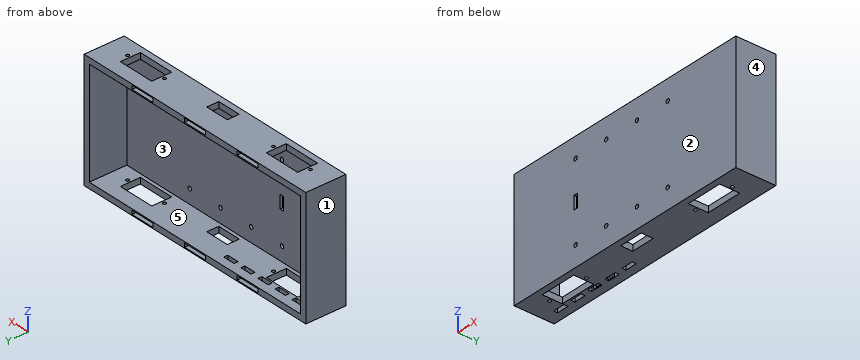
Autodesk Inventor part; units mm, degrees
ref_plane "Work Plane2" through (0, 19.05, 0) normal (0, 1, 0) x (1, 0, 0)
ref_plane "YZ Plane" through (0, 0, 0) normal (1, 0, 0) x (0, 1, 0)
ref_plane "XZ Plane" through (0, 0, 0) normal (0, 1, 0) x (-1, 0, 0)
sketch "Sketch1" plane through (0, 0, 0) normal (0, 1, 0) x (-1, 0, 0)
  line L0 (82.5, 37.5) -> (-82.5, 37.5)
  line L1 (-82.5, 37.5) -> (-82.5, -37.5)
  line L2 (-82.5, -37.5) -> (82.5, -37.5)
  line L3 (82.5, -37.5) -> (82.5, 37.5)
  point P0 (0, 0)
  point P1 (82.5, 0)
  point P2 (0, -37.5)
  dimension "d0" = 165
  dimension "d1" = 75
extrude "Extrusion1" add sketch "Sketch1" along normal blind 25.4
sketch "Sketch2" plane through (-82.5, 0, 37.5) normal (0, 0, 1) x (1, 0, 0)
  line L0 (39.878, 16.51) -> (16.51, 16.51)
  line L1 (39.878, 3.81) -> (39.878, 16.51)
  line L2 (16.51, 3.81) -> (39.878, 3.81)
  line L3 (16.51, 16.51) -> (16.51, 3.81)
  circle A0 centre (14.4272, 10.16) radius 1.016
  circle A1 centre (41.9608, 10.16) radius 1.016
  line L4 (0, 0) -> (165, 0)
  line L5 (0, 0) -> (0, 25.4)
  line L6 (148.49, 16.51) -> (125.122, 16.51)
  circle A2 centre (150.5728, 10.16) radius 1.016
  line L7 (148.49, 3.81) -> (148.49, 16.51)
  line L8 (125.122, 3.81) -> (148.49, 3.81)
  line L9 (125.122, 16.51) -> (125.122, 3.81)
  circle A3 centre (123.0392, 10.16) radius 1.016
  line L10 (165, 0) -> (165, 25.4)
  line L11 (74.88, 11.43) -> (90.12, 11.43)
  line L12 (90.12, 11.43) -> (90.12, 3.81)
  line L13 (90.12, 3.81) -> (74.88, 3.81)
  line L14 (74.88, 3.81) -> (74.88, 11.43)
  point P0 (82.5, 0)
  point P1 (16.51, 10.16)
  point P2 (39.878, 10.16)
  point P3 (0, 12.7)
  point P4 (125.122, 10.16)
  point P5 (82.5, 11.43)
  point P6 (82.5, 0)
  point P7 (74.88, 7.62)
  point P8 (148.49, 10.16)
  point P9 (90.12, 7.62)
  dimension "d4" = 12.7
  dimension "d5" = 23.368
  dimension "d6" = 2.032
  dimension "d7" = 2.032
  dimension "d8" = 2.0828
  dimension "d9" = 2.0828
  dimension "d11" = 16.51
  dimension "d12" = 12.7
  dimension "d13" = 23.368
  dimension "d14" = 2.032
  dimension "d15" = 2.032
  dimension "d16" = 2.0828
  dimension "d17" = 2.0828
  dimension "d18" = 16.51
  dimension "d19" = 15.24
  dimension "d20" = 7.62
  dimension "d55" = 10.16
  dimension "d56" = 10.16
  dimension "d58" = 7.62
extrude "Extrusion2" cut sketch "Sketch2" against normal blind 100.0125
sketch "Sketch3" plane through (0, 25.4, 0) normal (0, 1, 0) x (1, 0, 0)
  line L0 (-78.69, 33.69) -> (78.69, 33.69)
  line L1 (78.69, 33.69) -> (78.69, -33.69)
  line L2 (78.69, -33.69) -> (-78.69, -33.69)
  line L3 (-78.69, -33.69) -> (-78.69, 33.69)
  line L4 (82.5, -37.5) -> (82.5, 37.5)
  line L5 (-82.5, 37.5) -> (-82.5, -37.5)
  line L6 (82.5, 37.5) -> (-82.5, 37.5)
  line L7 (-82.5, -37.5) -> (82.5, -37.5)
  point P0 (0, 0)
  dimension "d25" = 3.81
  dimension "d26" = 3.81
  dimension "d27" = 3.81
  dimension "d28" = 3.81
extrude "Extrusion3" cut sketch "Sketch3" against normal blind 23.8125 contours L0 L1 L2 L3
sketch "Sketch4" plane through (0, 1.5875, 0) normal (0, 1, 0) x (1, 0, 0)
  circle A0 centre (31.7833, 24.6457) radius 1.27
  line L0 (-42.5, 20.5817) -> (42.5, 20.5817)
  circle A1 centre (8.9233, 24.6457) radius 1.27
  circle A2 centre (-13.9367, 24.6457) radius 1.27
  circle A3 centre (-36.7967, 24.6457) radius 1.27
  line L1 (67.3028, 0) -> (-67.3028, 0)
  circle A4 centre (31.7833, -24.6457) radius 1.27
  circle A5 centre (8.9233, -24.6457) radius 1.27
  circle A6 centre (-13.9367, -24.6457) radius 1.27
  circle A7 centre (-36.7967, -24.6457) radius 1.27
  line L2 (78.69, 33.69) -> (78.69, -33.69)
  line L3 (-38.0667, -4.2532) -> (-35.5267, -4.2532)
  line L4 (-35.5267, -4.2532) -> (-35.5267, 4.1493)
  line L5 (-35.5267, 4.1493) -> (-38.0667, 4.1493)
  line L6 (-38.0667, 4.1493) -> (-38.0667, -4.2532)
  point P0 (0, 0)
  point P1 (-11.4746, -1.9183)
  point P2 (78.69, 0)
  point P3 (0, 0)
  point P4 (0, 20.5817)
  point P5 (-36.7967, -4.2532)
  dimension "d35" = 2.54
  dimension "d36" = 4.064
  dimension "d37" = 22.86
  dimension "d159" = 20.3925
  dimension "d160" = 49.2914
extrude "Extrusion4" cut sketch "Sketch4" against normal blind 22.225
ref_plane "Work Plane2" through (0, 19.05, 0) normal (0, 1, 0) x (1, 0, 0)
sketch "Sketch9" plane through (0, 25.4, 0) normal (0, 1, 0) x (1, 0, 0)
  line L0 (-46.8649, 36.8624) -> (-31.3709, 36.8624)
  line L1 (-31.3709, 36.8624) -> (-31.3709, 34.452)
  line L2 (-31.3709, 34.452) -> (-46.8649, 34.452)
  line L3 (-46.8649, 34.452) -> (-46.8649, 36.8624)
  line L4 (31.3709, 36.8624) -> (46.8649, 36.8624)
  line L5 (46.8649, 36.8624) -> (46.8649, 34.452)
  line L6 (46.8649, 34.452) -> (31.3709, 34.452)
  line L7 (31.3709, 34.452) -> (31.3709, 36.8624)
  line L8 (-7.7489, 36.8624) -> (7.7489, 36.8624)
  line L9 (7.7489, 36.8624) -> (7.7489, 34.452)
  line L10 (7.7489, 34.452) -> (-7.7489, 34.452)
  line L11 (-7.7489, 34.452) -> (-7.7489, 36.8624)
  line L12 (82.5, -37.5) -> (82.5, 37.5)
  line L13 (-82.5, 37.5) -> (-82.5, -37.5)
  line L14 (-67.8534, 0) -> (73.4776, 0)
  line L15 (-46.8649, -36.8624) -> (-31.3709, -36.8624)
  line L16 (-31.3709, -36.8624) -> (-31.3709, -34.452)
  line L17 (-31.3709, -34.452) -> (-46.8649, -34.452)
  line L18 (-46.8649, -34.452) -> (-46.8649, -36.8624)
  line L19 (31.3709, -36.8624) -> (46.8649, -36.8624)
  line L20 (46.8649, -36.8624) -> (46.8649, -34.452)
  line L21 (46.8649, -34.452) -> (31.3709, -34.452)
  line L22 (31.3709, -34.452) -> (31.3709, -36.8624)
  line L23 (-7.7489, -36.8624) -> (7.7489, -36.8624)
  line L24 (7.7489, -36.8624) -> (7.7489, -34.452)
  line L25 (7.7489, -34.452) -> (-7.7489, -34.452)
  line L26 (-7.7489, -34.452) -> (-7.7489, -36.8624)
  line L27 (-78.69, 33.69) -> (78.69, 33.69)
  point P0 (0, 0)
  point P1 (-31.3709, 35.6572)
  point P2 (31.3709, 35.6572)
  point P3 (-7.7489, 35.6572)
  point P4 (7.7489, 35.6572)
  point P5 (0, 34.452)
  dimension "d59" = 2.4104
  dimension "d60" = 2.4104
  dimension "d61" = 2.4104
  dimension "d62" = 23.622
  dimension "d63" = 23.622
  dimension "d64" = 15.4979
  dimension "d65" = 15.494
  dimension "d66" = 15.494
  dimension "d85" = 0.762
extrude "Extrusion6" cut sketch "Sketch9" against normal blind 6.35
sketch "Sketch12" plane through (-78.69, 25.4, -33.69) normal (0, 0, 1) x (1, 0, 0)
  line L0 (5.08, -5.334) -> (12.7, -5.334)
  line L1 (12.7, -5.334) -> (12.7, -7.874)
  line L2 (12.7, -7.874) -> (5.08, -7.874)
  line L3 (5.08, -7.874) -> (5.08, -5.334)
  line L4 (0, 0) -> (157.38, 0)
  line L5 (0, 0) -> (0, -23.8125)
  line L6 (17.78, -5.334) -> (25.4, -5.334)
  line L7 (25.4, -5.334) -> (25.4, -7.874)
  line L8 (25.4, -7.874) -> (17.78, -7.874)
  line L9 (17.78, -7.874) -> (17.78, -5.334)
  line L10 (30.48, -5.334) -> (38.1, -5.334)
  line L11 (38.1, -5.334) -> (38.1, -7.874)
  line L12 (38.1, -7.874) -> (30.48, -7.874)
  line L13 (30.48, -7.874) -> (30.48, -5.334)
  line L14 (43.18, -5.334) -> (50.8, -5.334)
  line L15 (50.8, -5.334) -> (50.8, -7.874)
  line L16 (50.8, -7.874) -> (43.18, -7.874)
  line L17 (43.18, -7.874) -> (43.18, -5.334)
  line L18 (55.88, -5.334) -> (63.5, -5.334)
  line L19 (63.5, -5.334) -> (63.5, -7.874)
  line L20 (63.5, -7.874) -> (55.88, -7.874)
  line L21 (55.88, -7.874) -> (55.88, -5.334)
  point P0 (78.69, -25.4)
  dimension "d123" = 2.54
  dimension "d124" = 7.62
  dimension "d125" = 5.334
  dimension "d126" = 5.08
  dimension "d127" = 7.62
  dimension "d128" = 2.54
  dimension "d129" = 5.334
  dimension "d130" = 5.08
  dimension "d131" = 7.62
  dimension "d132" = 2.54
  dimension "d133" = 5.334
  dimension "d134" = 5.08
  dimension "d135" = 7.62
  dimension "d136" = 2.54
  dimension "d137" = 5.334
  dimension "d138" = 5.08
  dimension "d139" = 7.62
  dimension "d140" = 2.54
  dimension "d141" = 5.334
  dimension "d142" = 5.08
extrude "Extrusion9" cut sketch "Sketch12" against normal blind 5.715
properties part number "cuerpo3"
Source: CAD feature listing. Evaluate the final solid. Frame: model axes, mm. Face numbers are marked on the shaded views. A direction names the side the tool comes from. Coordinates: 2 decimals unless noted, no trailing zeros. Order: outer loops, then holes, each group sorted by start corner. A loop starts at its lowest first (then second) coordinate and runs counter-clockwise, first axis right, second up. Notation, with made-up numbers: (85, 4) - (123, 4) arc R15 ccw to (123, 33) - close; hole circle Ø3 at (30.5, 59.5). An arc over 180 degrees is marked (long way). One line per item, written item: value.
1) Cut plane B-B on y = 6.75. State how many separate pieces and enclosed holes the cut face has, plus the area to 3 significant figures.
Computed values:
separate pieces: 6
enclosed holes: 0
area: 1,300 mm^2
2) Contact query for flat-ended pins moving along their axis: pin 1 (20 mm diameter, centred on x = 1.5, z = 15.5, fed in from +Y); pin 2 (1.2 mm diameter, centred on x = -38, z = -35.5, fed in from +Y). Output: stop coordinate, or through.
Computed values:
pin 1: stops at y = 1.59
pin 2: stops at y = 19.05
3) Cut plane C-C on z = -11.5. Output: boundary loops of the cut face in (x, y).
Computed values:
outline: (-82.5, 0) - (82.5, 0) - (82.5, 25.4) - (78.69, 25.4) - (78.69, 1.59) - (-78.69, 1.59) - (-78.69, 25.4) - (-82.5, 25.4) - close
4) Reachability of the marked faces 4 and 5 from +Z, -Z, +X, -X, +Y, -Y: full face, straight path, thin tool, end or side. Return the list, or none.
Computed values:
face 4: +Z, -Z, +X, +Y, -Y
face 5: +Y
5) Cut plane A-A on y = 13.75. Output: boundary loops of the cut face in (x, z), plus the area to 3 significant figures.
Computed values:
outline: (-82.5, -37.5) - (-65.99, -37.5) - (-65.99, -33.69) - (-78.69, -33.69) - (-78.69, 33.69) - (-65.99, 33.69) - (-65.99, 37.5) - (-82.5, 37.5) - close; (-42.62, -37.5) - (42.62, -37.5) - (42.62, -33.69) - (-42.62, -33.69) - close; (-42.62, 33.69) - (42.62, 33.69) - (42.62, 37.5) - (-42.62, 37.5) - close; (65.99, -37.5) - (82.5, -37.5) - (82.5, 37.5) - (65.99, 37.5) - (65.99, 33.69) - (78.69, 33.69) - (78.69, -33.69) - (65.99, -33.69) - close
area: 1,410 mm^2
6) Ray query, line 1 (Z direction, x = -6.5, y = 19.25); line 2 (X direction, y = 15.75, z = 34.5); line 3 (X direction, y = 9.25, z = 2). Return the intervals inside material, ascending. Write a range as [from, to].
Computed values:
line 1: z = [-37.5, -36.86], [-34.45, -33.69], [33.69, 34.45], [36.86, 37.5]
line 2: x = [-82.5, -65.99], [-42.62, 42.62], [65.99, 82.5]
line 3: x = [-82.5, -78.69], [78.69, 82.5]
7) Mould query, pull axis X, two halves, no side actions, for the marked faces 1, 2 and 3. Classes: released by +X, released by -X, zero draft, split by the parting line, or undercut.
Computed values:
face 1: released by -X
face 2: zero draft
face 3: undercut
